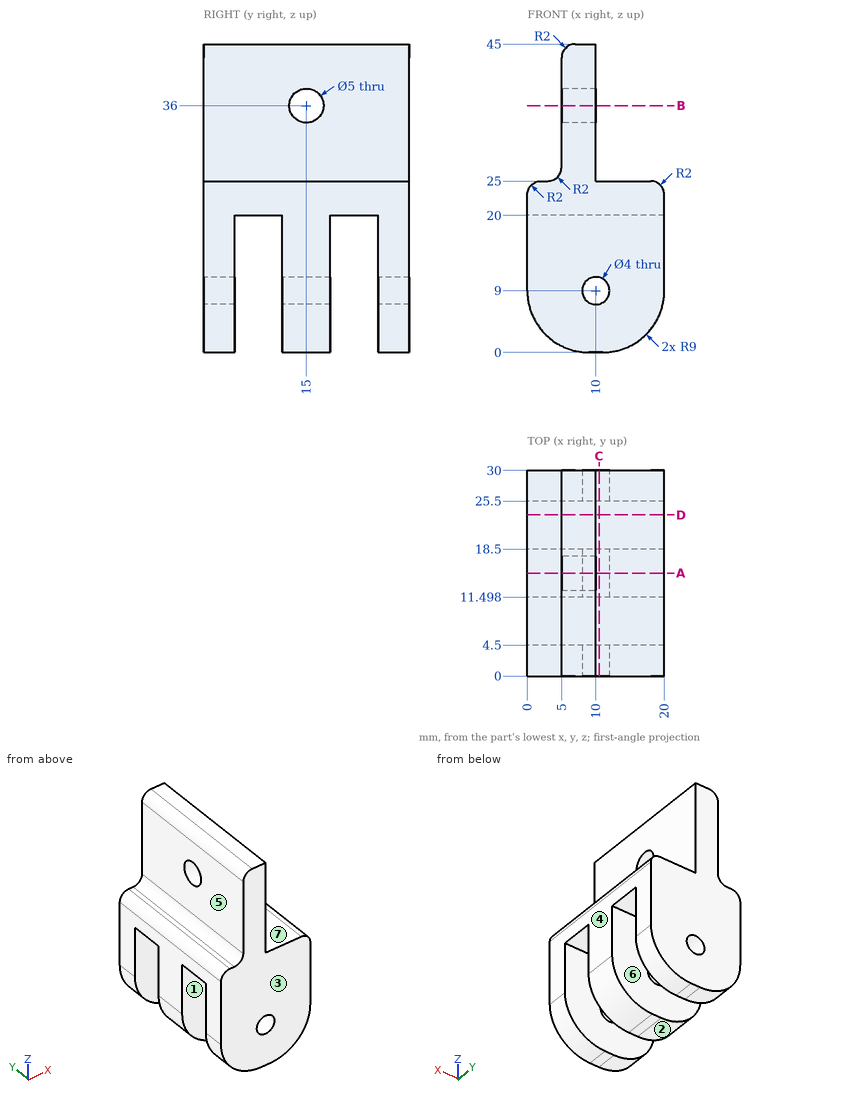
Geometry check sheet. Reference: drawing and pictorial views, mm from the part's lowest x, y, z. A direction names the side the tool comes from. Give positions to 0.01 mm unless a question says otherwise; leave off trailing zeros. Loops run counter-clockwise (first coordinate to the right, second up) from the corner with the lowest first, then second, coordinate; pieces in that order, holes last.
1. Go/stop test with flat-tipped pins: pin 1 Ø4 at (y, z) = (9, 29.5) entering from +X; pin 2 Ø3.5 at (x, y) = (8, 23.5) entering from -Z; pin 3 Ø7.5 at (x, y) = (5.5, 9) entering from -Z. Record where each tip stops, or that it passes through.
2. Section check B-B, the plane z = 36. Enter the section's corners in (x, y).
3. Set-up check for the marked faces 4, 5, 6 and 7: record each of +Z, -Z, +X, -X, +Y, -Y from which the full face is reachable in a straight line by a thin tool's end or side.
4. Section check C-C, the plane x = 10.5. Enter the section's corners in (y, z), then the cut area to 3 significant figures.
5. Mould release check, pull along Y, two halves, no side actions. Record for the marked faces 1, 2 and 3: released by +Y, released by -Y, zero draft, split by the parting line, or undercut.
6. Thickness scan on line 1 (Y direction, x = 13.5, z = 10); line 2 (Z direction, x = 8.65, y = 15) (1 decimal); line 3 (X direction, y = 1.5, z = 35). Record the ranges inside material, lowest first.
7. Section check A-A, the plane y = 15. Enter the section's corners in (x, z).
8. Section check D-D, the plane y = 23.5. Enter the section's corners in (x, z), then the cut area to 3 significant figures.
Geometry says:
1. pin 1: stops at x = 10
1. pin 2: stops at z = 20
1. pin 3: stops at z = 0.03
2. outline: (5, 0) - (10, 0) - (10, 12.5) - (5, 12.5) - close; (5, 17.5) - (10, 17.5) - (10, 30) - (5, 30) - close
3. face 4: +Z, -Z, +X, +Y, -Y
3. face 5: +Z, -X, +Y, -Y
3. face 6: -Z, +X, -X
3. face 7: +Z, +X, +Y, -Y
4. outline: (0, 0) - (4.5, 0) - (4.5, 7.06) - (0, 7.06) - close; (0, 10.94) - (4.5, 10.94) - (4.5, 20) - (11.5, 20) - (11.5, 10.94) - (18.5, 10.94) - (18.5, 20) - (25.5, 20) - (25.5, 10.94) - (30, 10.94) - (30, 25) - (0, 25) - close; (11.5, 0) - (18.5, 0) - (18.5, 7.06) - (11.5, 7.06) - close; (25.5, 0) - (30, 0) - (30, 7.06) - (25.5, 7.06) - close
4. area: 408 mm2
5. face 1: undercut
5. face 2: zero draft
5. face 3: released by -Y
6. line 1: y = 0 to 4.5, 11.5 to 18.5, 25.5 to 30
6. line 2: z = 0 to 7.5, 10.5 to 33.5, 38.5 to 45
6. line 3: x = 5 to 10
7. outline: (0, 9) arc R9 ccw to (9, 0) - (11, 0) arc R9 ccw to (20, 9) - (20, 23) arc R2 ccw to (18, 25) - (10, 25) - (10, 33.5) - (5, 33.5) - (5, 27) arc R2 cw to (3, 25) - (2, 25) arc R2 ccw to (0, 23) - close; (5, 38.5) - (10, 38.5) - (10, 45) - (7, 45) arc R2 ccw to (5, 43) - close; hole circle Ø4 at (10, 9)
8. outline: (0, 20) - (20, 20) - (20, 23) arc R2 ccw to (18, 25) - (10, 25) - (10, 45) - (7, 45) arc R2 ccw to (5, 43) - (5, 27) arc R2 cw to (3, 25) - (2, 25) arc R2 ccw to (0, 23) - close
8. area: 198 mm2
